from build123d import *

# Parameters (mm, degrees)
SKETCH1_W               = 8
SKETCH1_H               = 8
BOSS_EXTRUDE1_DEPTH     = 3
CUT_EXTRUDE1_DEPTH      = 12.704699911
CUT_EXTRUDE1_DEPTH_BACK = 12.704699911
CUT_EXTRUDE2_DEPTH      = 11
SKETCH4_R               = 1.8
CUT_EXTRUDE3_DEPTH      = 0.8
SKETCH5_W               = 8
SKETCH5_H               = 1
BOSS_EXTRUDE2_DEPTH     = 2
FILLET1_R               = 4
SKETCH6_W               = 2.10217216
SKETCH6_H               = 1.6
CUT_EXTRUDE4_DEPTH      = 0.4


with BuildPart() as part:
    # Sketch1 → Boss-Extrude1 (new body)
    with BuildSketch(Plane(origin=(0, 0, 0), x_dir=(1, 0, 0), z_dir=(0, 1, 0))):
        with Locations((4, 4)):
            Rectangle(SKETCH1_W, SKETCH1_H)
    extrude(amount=BOSS_EXTRUDE1_DEPTH)

    # Sketch2 → Cut-Extrude1 (cut, two sides: drawn at the far end of the back side and taken through both)
    with BuildSketch(Plane.XY.offset(-CUT_EXTRUDE1_DEPTH_BACK)):
        Polygon((0, 0), (0.6, 3), (0, 3), align=None)
        Polygon((8, 0), (7.4, 3), (8, 3), align=None)
    extrude(amount=CUT_EXTRUDE1_DEPTH + CUT_EXTRUDE1_DEPTH_BACK, mode=Mode.SUBTRACT)

    # Sketch3 → Cut-Extrude2 (cut)
    with BuildSketch(Plane(origin=(0, 0, 0), x_dir=(0, 0, -1), z_dir=(1, 0, 0))):
        Polygon((0, 0), (0.6, 3), (0, 3), align=None)
        Polygon((8, 3), (7.4, 3), (8, 0), align=None)
    extrude(amount=CUT_EXTRUDE2_DEPTH, mode=Mode.SUBTRACT)

    # Sketch4 → Cut-Extrude3 (cut)
    with BuildSketch(Plane.XZ):
        with Locations(Location((4, -3.75, 0), (0, 0, 270))):
            Circle(SKETCH4_R)
    extrude(amount=-CUT_EXTRUDE3_DEPTH, mode=Mode.SUBTRACT)

    # Sketch5 → Boss-Extrude2 (add)
    with BuildSketch(Plane.XZ):
        with Locations((4, -7.5)):
            Rectangle(SKETCH5_W, SKETCH5_H)
    extrude(amount=BOSS_EXTRUDE2_DEPTH)

    # Fillet1
    # the kernel refuses this fillet: 4 mm, written as the material it takes off along each edge
    with BuildSketch(Plane(origin=(8, -2, -16.660254038), x_dir=(0, 1, 0), z_dir=(0, 0, 1)), Plane(origin=(0, -2, 1.660254038), x_dir=(0, 1, 0), z_dir=(0, 0, -1))) as fillet1_piece_1:
        with BuildLine():
            CenterArc((4, 3.464101615), FILLET1_R, 180, 60)
            Line((0, 3.464101615), (-0.08, 3.464101615))
            Line((-0.08, 3.464101615), (-0.08, 0))
            Line((-0.08, 0), (0, -0.08))
            ThreePointArc((0, -0.08), (1, -0.08), (1.96, -0.069282032))
            Line((1.96, -0.069282032), (2, 0))
        make_face()
    extrude(amount=18.320508076, mode=Mode.SUBTRACT)

    # Sketch6 → Cut-Extrude4 (cut)
    with BuildSketch(Plane(origin=(0, 3, 0), x_dir=(1, 0, 0), z_dir=(0, 1, 0))):
        Polygon((3.09782784, 2.1), (3.09782784, 3.7), (3.09782784, 4.7), (1.1, 2.9), (3.09782784, 1.1), align=None)
        with Locations((4.14891392, 2.9)):
            Rectangle(SKETCH6_W, SKETCH6_H)
        Polygon((5.2, 6.8), (5.2, 3.7), (5.2, 2.1), (6.8, 2.1), (6.8, 6.8), align=None)
    extrude(amount=-CUT_EXTRUDE4_DEPTH, mode=Mode.SUBTRACT)


solid = part.part
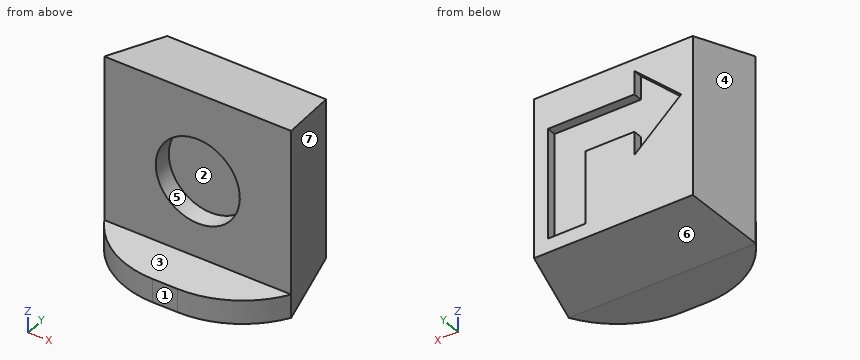
Model file for the job. Use its own axes, mm. Face numbers are marked on the shaded views. A direction names the side the tool comes from. Round coordinates to 2 decimals unless told otherwise and drop trailing zeros. Order: outer loops, then holes, each group sorted by start corner. A loop starts at its lowest first (then second) coordinate and runs counter-clockwise, first axis right, second up. Notation, with made-up numbers: M 28,82 L 77,82 A19 ccw 77,104 Z; hole C 9,36.5 d1. An arc over 180 degrees is marked long. Write each question's results on one line, items separated by ' | '. Start each with the question number.
(1) Saw through at B-B, the plane x = 4. Give the cut face in (y, z), then the cut area to 3 significant figures.
(2) Probe probe 1 along Y at (x, z) = (1, -6); probe 2 along Z at (x, y) = (5.75, -0.05); probe 3 along Y at (x, z) = (3, -1.5). List the from-to ranges inside material, lowest first. Write a range as from..to.
(3) Saw through at A-A, the plane y = 0.5. Give the cut face in (x, z).
(4) Drop flat-ended pins along their axis: pin 1 (4 mm diameter, centred on x = 4.5, z = -4.5, fed in from -Y); pin 2 (2 mm diameter, centred on y = 1.5, z = -5, fed in from +X); pin 3 (1.5 mm diameter, centred on x = 5.5, y = 1.5, fed in from -Z). Give the stop position or say it passes through.
(5) Two-plate mould, pull along X, no slides. Class the marked faces 4, 5, 6 and 7: pulls with the +X half, pulls with the -X half, needs draft (parallel to the pull), parting line crosses it, or undercut.
(6) Saw through at C-C, the plane z = -7.25. Give the cut face in (x, y).
(7) Saw through at D-D, the plane y = 1.45. Give the cut face in (x, z).
(8) Which spindle directions (+Z, -Z, +X, -X, +Y, -Y) get a long thin tool onto all of the face, cutting with end or side? Do the marked faces 1, 2 and 3. Say none if no direction does.
Established:
1) outline: M -2,-8 L 0,-8 L 3,-7.4 L 3,-3.7 L 2.6,-3.7 L 2.6,-2.1 L 3,-2.1 L 3,-0.6 L 0,0 L 0,-1.95 L 0.8,-1.95 L 0.8,-5.55 L 0,-5.55 L 0,-7 L -2,-7 Z | area: 20.7 mm^2
2) probe 1: y = 0..3 | probe 2: z = -8..-7 | probe 3: y = 0..2.6
3) outline: M 0.1,-7.9 L 7.9,-7.9 L 7.9,-0.1 L 0.1,-0.1 Z; hole C 4,-3.75 d3.6
4) pin 1: stops at y = 0 | pin 2: stops at x = 7.9 | pin 3: stops at z = -7.85
5) face 4: pulls with the -X half | face 5: undercut | face 6: needs draft | face 7: pulls with the +X half
6) outline: M 0,0 A4 ccw 3.46,-2 L 4.54,-2 A4 ccw 8,0 L 7.4,3 L 0.6,3 Z
7) outline: M 0.29,-7.71 L 7.71,-7.71 L 7.71,-0.29 L 0.29,-0.29 Z
8) face 1: +Z, -Z, +X, -X, -Y | face 2: -Y | face 3: +Z, +X, -X, -Y
